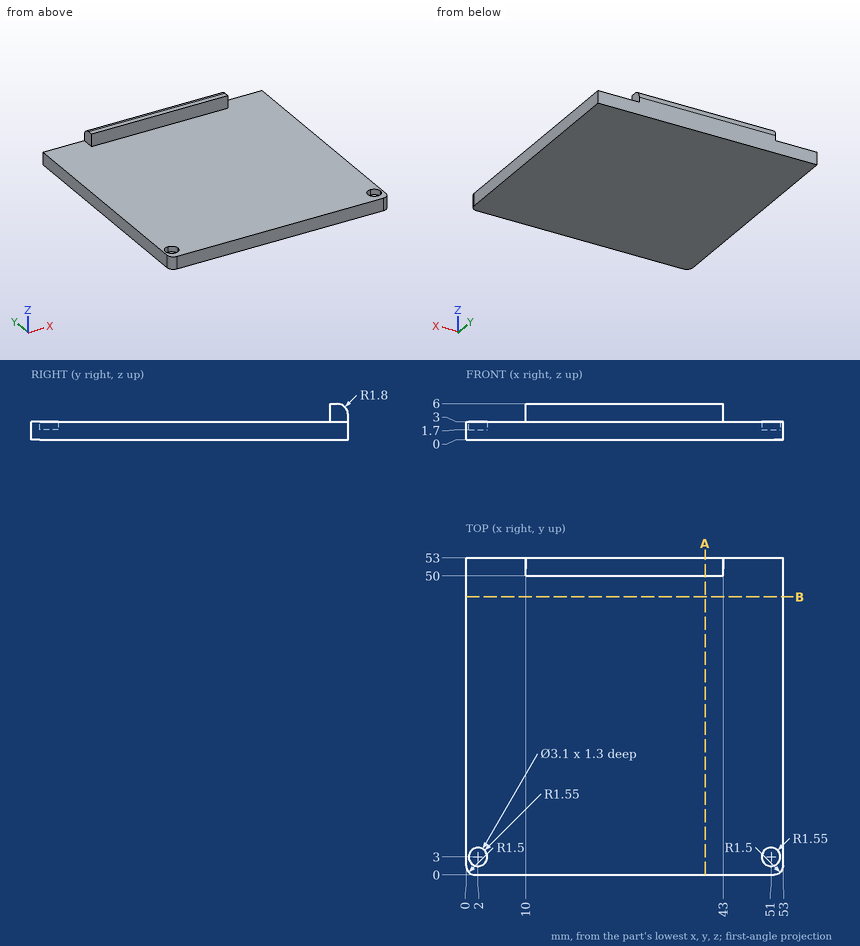
Source: three-view drawing plus pictorial views. Frame: mm from the lowest corner of the part. Round coordinates to 2 decimals unless told otherwise and drop trailing zeros. Loops run counter-clockwise (first coordinate to the right, second up) from the corner with the lowest first, then second, coordinate; pieces in that order, holes last.
Q1. Section B-B, the plane y = 46.5. Return loops of the section in (x, z).
Q2. Ray query, line 1 (X direction, y = 3, z = 2.3); line 2 (Y direction, x = 2, z = 2.65); line 3 (Z direction, x = 39, y = 13). Return the intervals inside material, ascending.
Q3. First-contact query: P1, Ø3, axis at x = 2, y = 3, coming from the +Z side; P2, Ø3.5, axis at x = 2.5, y = 2.5, coming from the +Z side; P3, Ø1.5, axis at x = 25, z = 5, coming from the -Y side. Flat tips, straight axial feed; report the tip coordinate or a pass-through.
Q4. Section A-A, the plane x = 40. Return loops of the section in (y, z), plus the area to 3 significant figures.
Solutions:
1. outline: (0, 0) - (53, 0) - (53, 3) - (0, 3) - close
2. line 1: x = 0 to 0.45, 3.55 to 49.45, 52.55 to 53
2. line 2: y = 0 to 1.45, 4.55 to 53
2. line 3: z = 0 to 3
3. P1: stops at z = 1.7
3. P2: stops at z = 3
3. P3: stops at y = 50
4. outline: (0, 0) - (53, 0) - (53, 4.2) arc R1.8 ccw to (51.2, 6) - (50, 6) - (50, 3) - (0, 3) - close
4. area: 167 mm2
